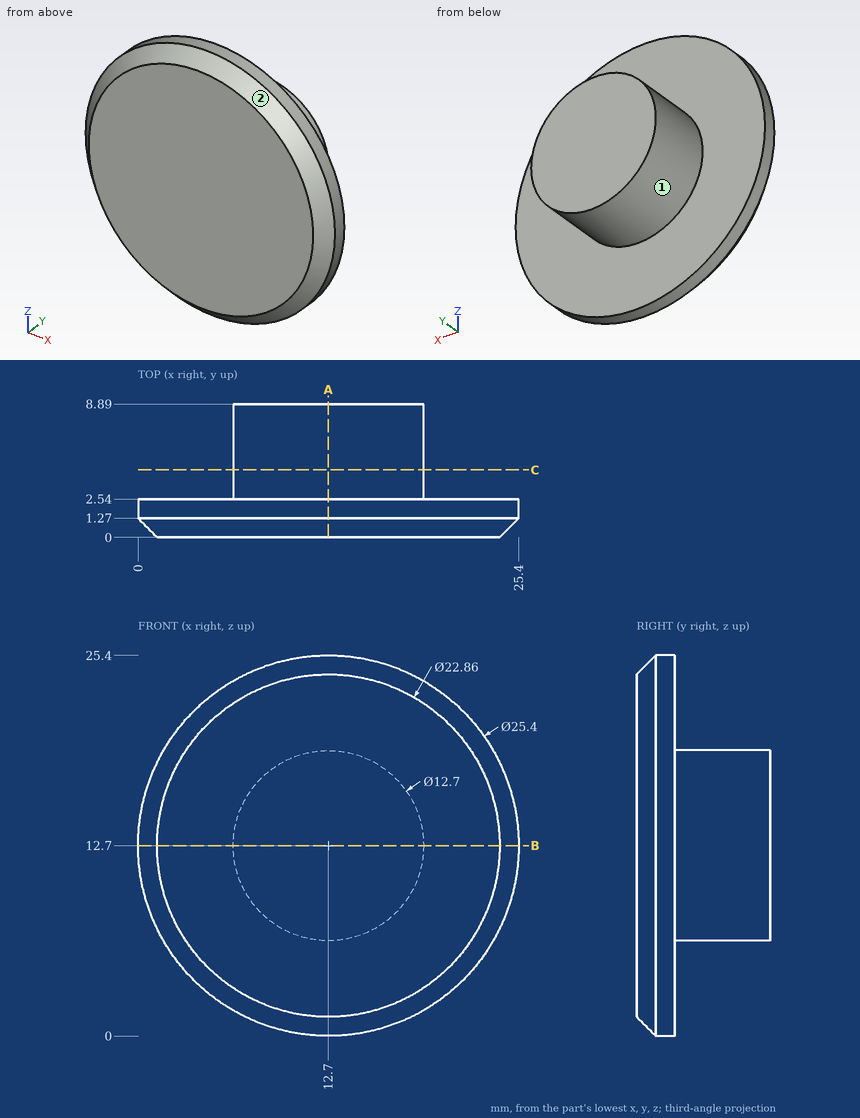
Can you work these out from the drawing? Everything is in mm from the part's minimum corner. A direction names the side the tool comes from. Round coordinates to 2 decimals unless told otherwise and drop trailing zeros. Order: outer loops, then holes, each group sorted by start corner. A loop starts at its lowest first (then second) coordinate and runs counter-clockwise, first axis right, second up. Notation, with made-up numbers: (53.25, 85.5) -> (106.25, 85.5) arc R34 ccw to (106.25, 119.5) -> close; hole circle Ø8 at (-33, -14). An arc over 180 degrees is marked (long way). Use CSV: the item, a comma, the result in double quotes.
1. I want a section at C-C on y = 4.5. List the corners of the cut face in (x, z) for me.
Recorded:
outline,"circle Ø12.7 at (12.7, 12.7)"
2. I want a section at B-B on z = 12.7. List the corners of the cut face in (x, y) for me, and give its area (3 significant figures).
Recorded:
outline,"(0, 1.27) -> (1.27, 0) -> (24.13, 0) -> (25.4, 1.27) -> (25.4, 2.54) -> (19.05, 2.54) -> (19.05, 8.89) -> (6.35, 8.89) -> (6.35, 2.54) -> (0, 2.54) -> close"
area,"144 mm2"
3. I'm going to push flat-ended pins straight in: P1, Ø4, axis at x = 18.5, y = 3, coming from the -Z side; P2, Ø5, axis at x = 8, y = 3.5, coming from the -Z side; P3, Ø2, axis at x = 5.5, y = 2.5, coming from the -Z side. Where does each tip first touch, or does it pass through?
Recorded:
P1,"stops at z = 0.6"
P2,"stops at z = 0.23"
P3,"stops at z = 1.62"
4. I need wall thicknesses on line 1 along Y through (x, z) = (20.5, 6.75); line 2 along Z through (x, y) = (7.75, 8); line 3 along Z through (x, y) = (10.5, 1). Which ranges of each line are inside material? Lowest first, please.
Recorded:
line 1,"y = 0 to 2.54"
line 2,"z = 8.72 to 16.68"
line 3,"z = 0.47 to 24.93"
5. Which directions (+Z, -Z, +X, -X, +Y, -Y) give clear straight access to the entire face, cutting with the end or side of a thin tool? Please do the marked faces 1 and 2.
Recorded:
face 1,"+Y"
face 2,"-Y"
6. I want a section at A-A on x = 12.7. List the corners of the cut face in (y, z) for me, and give its area (3 significant figures).
Recorded:
outline,"(0, 1.27) -> (1.27, 0) -> (2.54, 0) -> (2.54, 6.35) -> (8.89, 6.35) -> (8.89, 19.05) -> (2.54, 19.05) -> (2.54, 25.4) -> (1.27, 25.4) -> (0, 24.13) -> close"
area,"144 mm2"
